Geometry: final body of the model. Coordinates: model frame, mm. A direction names the side the tool comes from. Round coordinates to 2 decimals unless told otherwise and drop trailing zeros. Loops run counter-clockwise (first coordinate to the right, second up) from the corner with the lowest first, then second, coordinate; pieces in that order, holes last. Notation, with made-up numbers: M 54,-21.75 L 72,-21.75 A16 cw 72,3.25 Z; hole C 87,0 d9. An arc over 180 degrees is marked long. Answer as a JSON object with one key per item and string values.
Autodesk Inventor part; units mm, degrees
ref_plane "YZ Plane" through (0, 0, 0) normal (1, 0, 0) x (0, 1, 0)
ref_plane "XZ Plane" through (0, 0, 0) normal (0, 1, 0) x (-1, 0, 0)
ref_plane "XY Plane" through (0, 0, 0) normal (0, 0, 1) x (1, 0, 0)
sketch "Sketch1" plane through (0, 0, 0) normal (0, 0, 1) x (1, 0, 0)
  line L0 (-38.3761, 21.7949) -> (114.0239, 21.7949)
  line L1 (114.0239, 21.7949) -> (114.0239, -79.8051)
  line L2 (114.0239, -79.8051) -> (-38.3761, -79.8051)
  line L3 (-38.3761, -79.8051) -> (-38.3761, 21.7949)
  dimension "d0" = 152.4
  dimension "d1" = 101.6
extrude "Extrusion1" add sketch "Sketch1" along normal blind 6.35
sketch "Sketch2" plane through (0, 0, 6.35) normal (0, 0, 1) x (1, 0, 0)
  line L0 (-38.3761, -79.8051) -> (-38.3761, 21.7949)
  line L1 (114.0239, -79.8051) -> (-38.3761, -79.8051)
  circle A0 centre (-25.6761, -67.1051) radius 3.81
  dimension "d4" = 7.62
  dimension "d5" = 12.7
  dimension "d6" = 12.7
extrude "Extrusion2" add sketch "Sketch2" along normal blind 6.35
pattern_linear "Rectangular Pattern1" count 6 spacing 25.4 along (1, 0, 0) count 4 spacing 25.4 along (0, 1, 0) of "Extrusion2"
properties part number "Rectangular"
1) Section query D-D (x = 49). Return the cut outline in (y, z), and give its area (3 significant figures).
Results:
{"outline": "M -79.81,0 L 21.79,0 L 21.79,6.35 L 12.59,6.35 L 12.59,12.7 L 5.6,12.7 L 5.6,6.35 L -12.81,6.35 L -12.81,12.7 L -19.8,12.7 L -19.8,6.35 L -38.21,6.35 L -38.21,12.7 L -45.2,12.7 L -45.2,6.35 L -63.61,6.35 L -63.61,12.7 L -70.6,12.7 L -70.6,6.35 L -79.81,6.35 Z", "area": "823 mm2"}
2) Section query B-B (x = 25.5). Return the cut outline in (y, z), and give its area (3 significant figures).
Results:
{"outline": "M -79.81,0 L 21.79,0 L 21.79,6.35 L 12.89,6.35 L 12.89,12.7 L 5.3,12.7 L 5.3,6.35 L -12.51,6.35 L -12.51,12.7 L -20.1,12.7 L -20.1,6.35 L -37.91,6.35 L -37.91,12.7 L -45.5,12.7 L -45.5,6.35 L -63.31,6.35 L -63.31,12.7 L -70.9,12.7 L -70.9,6.35 L -79.81,6.35 Z", "area": "838 mm2"}
3) Section query C-C (y = 11). Return the cut outline in (x, z).
Results:
{"outline": "M -38.38,0 L 114.02,0 L 114.02,6.35 L 104.62,6.35 L 104.62,12.7 L 98.02,12.7 L 98.02,6.35 L 79.22,6.35 L 79.22,12.7 L 72.62,12.7 L 72.62,6.35 L 53.82,6.35 L 53.82,12.7 L 47.22,12.7 L 47.22,6.35 L 28.42,6.35 L 28.42,12.7 L 21.82,12.7 L 21.82,6.35 L 3.02,6.35 L 3.02,12.7 L -3.58,12.7 L -3.58,6.35 L -22.38,6.35 L -22.38,12.7 L -28.98,12.7 L -28.98,6.35 L -38.38,6.35 Z"}
4) Pin query (flat end, axial travel): P1, Ø1, axis at x = 49, z = 8, coming from the -Y side. Return the tip coordinate at first contact, or that it passes through.
Results:
{"P1": "y = -70.77"}
5) Pull-direction query (X, two-part tool) for faces 1 (the flat face through (76, -67, 12.7)), 2 (the flat face through (114.024, -28, 3)), 3 (the cylindrical face through (49.698, -63.386, 9.481)); classes: +X half, -X half, draft (parallel to the pull), parting line (faces both ways), or undercut.
Results:
{"face 1": "draft", "face 2": "+X half", "face 3": "undercut"}
6) Reachability of faces 4 (the flat face through (25, -67, 12.7)), 5 (the cylindrical face through (-29.482, -16.473, 9.481)) from +Z, -Z, +X, -X, +Y, -Y: full face, straight path, thin tool, end or side. Return the list, or none.
Results:
{"face 4": "+Z, +X, -X, +Y, -Y", "face 5": "+Z"}
7) Ray query, line 1 (X direction, y = -39, z = 9.25); line 2 (Y direction, x = 52.5, z = 11.75); line 3 (Y direction, x = 48, z = 10). Return the intervals inside material, ascending.
Results:
{"line 1": "-28.36 to -22.99, -2.96 to 2.41, 22.44 to 27.81, 47.84 to 53.21, 73.24 to 78.61, 98.64 to 104.01", "line 2": "-70.36 to -63.85, -44.96 to -38.45, -19.56 to -13.05, 5.84 to 12.35", "line 3": "-69.96 to -64.25, -44.56 to -38.85, -19.16 to -13.45, 6.24 to 11.95"}
8) Section query A-A (z = 11). Count the separate pieces of the cut face and the enclosed holes in it, and give its area (3 significant figures).
Results:
{"separate pieces": "24", "enclosed holes": "0", "area": "1,090 mm2"}
